Source: CAD feature listing. Evaluate the final solid. Frame: model axes, mm. Face numbers are marked on the shaded views. Round coordinates to 2 decimals unless told otherwise and drop trailing zeros. Write item = value, one per line. Start each with the question number.
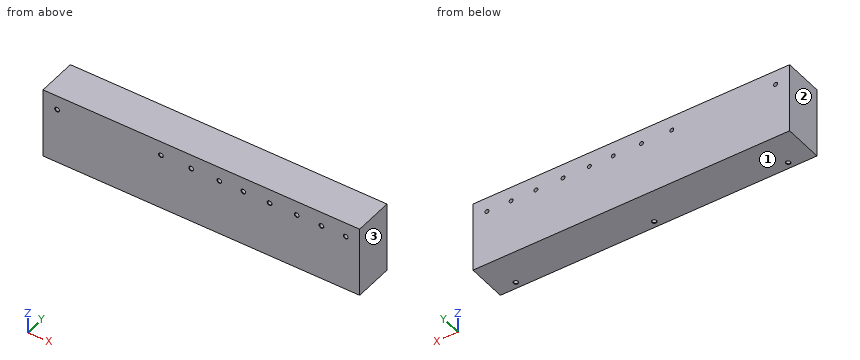
from build123d import *

# Parameters (mm, degrees)
F0_W           = 200.0950425863
F0_H           = 44.5620156825
F1_DEPTH       = 25
F3_D           = 2.5
F3_CSINK_D     = 3
F3_CSINK_ANGLE = 90
F5_D           = 2.5
F5_DEPTH       = 15
F5_CSINK_D     = 3
F5_CSINK_ANGLE = 90
F5_TIP         = 0.7510757738


with BuildPart() as f1:
    # F0 (on Front) → F1 (new body)
    with BuildSketch(Plane.XZ):
        Rectangle(F0_W, F0_H)
    extrude(amount=F1_DEPTH)

    # F3 (through all)
    with Locations(Plane.XZ.offset(25)):
        with Locations((-91.1486074328, 13.1441922858), (-25.5451947451, 13.1441922858), (-6.4415293746, 13.1441922858), (11.4006157964, 13.1441922858), (26.5406873077, 13.1441922858), (43.1231148541, 13.1441922858), (60.2437853813, 13.1441922858), (75.9239122272, 13.1441922858), (91.2448167801, 13.1441922858)):
            CounterSinkHole(F3_D / 2, F3_CSINK_D / 2, counter_sink_angle=F3_CSINK_ANGLE)

    # F5
    with Locations(Plane(origin=(0, 0, -22.2810078412), x_dir=(1, 0, 0), z_dir=(0, 0, -1))):
        with Locations((87.427444756, 20.9353156388), (0, 20.9353156388), (-84.652133286, 20.9353156388)):
            CounterSinkHole(F5_D / 2, F5_CSINK_D / 2, depth=F5_DEPTH, counter_sink_angle=F5_CSINK_ANGLE)
            with Locations((0, 0, -(F5_DEPTH + F5_TIP / 2))):  # 118° drill point
                Cone(0, F5_D / 2, F5_TIP, mode=Mode.SUBTRACT)


solid = f1.part
(1) Material intervals for line 1 along Z through (x, y) = (42, -2); line 2 along Z through (x, y) = (42.5, -8); line 3 along Z through (x, y) = (0.5, -21.5), sorted ascending. Write a range as from..to.
(2) Mould query, pull axis X, two halves, no side actions, for the marked faces 1, 2 and 3. Classes: +X half, -X half, draft (parallel to the pull), parting line (faces both ways), or undercut.
(3) Pin query (flat end, axial travel): P1, Ø1.5, axis at x = 87.43, y = -20.94, coming from the -Z side. Return the tip coordinate at first contact, or that it passes through.
Solution:
q1.line_1 = -22.28..12.6, 13.69..22.28
q1.line_2 = -22.28..12.06, 14.23..22.28
q1.line_3 = -6.98..22.28
q2.face_1 = draft
q2.face_2 = -X half
q2.face_3 = +X half
q3.P1 = -6.98
